Geometry: final body of the model. Coordinates: model frame, mm. A direction names the side the tool comes from. Round coordinates to 2 decimals unless told otherwise and drop trailing zeros. Order: outer loops, then holes, each group sorted by start corner. A loop starts at its lowest first (then second) coordinate and runs counter-clockwise, first axis right, second up. Notation, with made-up numbers: (89.25, -31.75) - (147.25, -31.75) arc R15 ccw to (147.25, -5.75) - close; hole circle Ø6 at (0, 19). An arc over 180 degrees is marked (long way). Put each result on its own line as item: value. Start each with the question number.
(1) Section A-A (z = 217.5). Output: boundary loops of the cut face in (x, y), and give its area (3 significant figures).
(2) Material intervals for L1, parallel to X at y = -137.5, z = 223.5; L2, parallel to Z at x = 28.5, y = 45.5; L3, parallel to Y at x = 349, z = 219.5, sorted ascending. Write a range as [from, to].
(3) Section B-B (x = 484). Output: boundary loops of the cut face in (y, z).
(4) Pin query (flat end, axial travel): P1, Ø8, axis at x = 383, z = 131.5, coming from the -Y side. Return the tip coordinate at first contact, or that it passes through.
(5) Access query for faces 5 (the face through (-239.349, -94, 177)), 6 (the face through (480, 48.507, 182)). Directions: +Z, -Z, +X, -X, +Y, -Y. A direction counts if a zero-diameter tool reaches every point of the face in a straight line with its end or side. Return the directions, or none.
(6) Section C-C (y = -123.5). Output: boundary loops of the cut face in (x, z).
(7) Pull-direction query (Z, two-part tool) for faces 1 (the face through (239, -89, 0)), 2 (the face through (239, -89, 360)), 3 (the face through (239, 58.507, 177)), 4 (the face through (5, -99, 340)); classes: released by +Z, released by -Z, zero draft, split by the parting line, or undercut.
from build123d import *

# Parameters (mm, degrees)
F0_W     = 970
F0_H     = 300
F1_DEPTH = 360
F2_W     = 455
F2_H     = 320
F3_DEPTH = 290
F4_W     = 455
F4_H     = 320
F5_DEPTH = 290


with BuildPart() as f1:
    # F0 (on Top) → F1 (new body)
    with BuildSketch(Plane.XY):
        with Locations((245.651422, -91.493237)):
            Rectangle(F0_W, F0_H)
    extrude(amount=F1_DEPTH)

    # F2 (on face) → F3 (cut)
    with BuildSketch(Plane.XZ.offset(241.493237)):
        with Locations((8.151422, 180)):
            Rectangle(F2_W, F2_H)
    extrude(amount=-F3_DEPTH, mode=Mode.SUBTRACT)

    # F4 (on face) → F5 (cut)
    with BuildSketch(Plane.XZ.offset(241.493237)):
        with Locations((483.151422, 180)):
            Rectangle(F4_W, F4_H)
    extrude(amount=-F5_DEPTH, mode=Mode.SUBTRACT)


solid = f1.part
Checks:
1. outline: (-239.35, -241.49) - (-219.35, -241.49) - (-219.35, 48.51) - (235.65, 48.51) - (235.65, -241.49) - (255.65, -241.49) - (255.65, 48.51) - (710.65, 48.51) - (710.65, -241.49) - (730.65, -241.49) - (730.65, 58.51) - (-239.35, 58.51) - close
1. area: 27,100 mm²
2. L1: x = [-239.35, -219.35], [235.65, 255.65], [710.65, 730.65]
2. L2: z = [0, 20], [340, 360]
2. L3: y = [48.51, 58.51]
3. outline: (-241.49, 0) - (58.51, 0) - (58.51, 360) - (-241.49, 360) - (-241.49, 340) - (48.51, 340) - (48.51, 20) - (-241.49, 20) - close
4. P1: stops at y = 48.51
5. face 5: +Z, -Z, -X, +Y, -Y
5. face 6: -Y
6. outline: (-239.35, 0) - (730.65, 0) - (730.65, 360) - (-239.35, 360) - close; hole (-219.35, 20) - (235.65, 20) - (235.65, 340) - (-219.35, 340) - close; hole (255.65, 20) - (710.65, 20) - (710.65, 340) - (255.65, 340) - close
7. face 1: released by -Z
7. face 2: released by +Z
7. face 3: zero draft
7. face 4: undercut
